Design review of the part built by this model. Coordinates are the model's own, in mm. A direction names the side the tool comes from. Coordinates: 2 decimals unless noted, no trailing zeros. Order: outer loops, then holes, each group sorted by start corner. A loop starts at its lowest first (then second) coordinate and runs counter-clockwise, first axis right, second up. Notation, with made-up numbers: M 24,-40 L 51,-40 A14 cw 51,-35 Z; hole C -11,-17 d10. An arc over 180 degrees is marked long. Answer as a JSON object with one key per item and string values.
from build123d import *

# Parameters (mm, degrees)
SKETCH1_W           = 66
SKETCH1_H           = 180
BOSS_EXTRUDE1_DEPTH = 34.7
FILLET1_R           = 10
SHELL1_T            = -3.1
SKETCH4_R           = 6.5
CUT_EXTRUDE4_DEPTH  = 35.7
SKETCH2_R           = 3.25
CUT_EXTRUDE5_DEPTH  = 35.7
SKETCH5_W           = 27
SKETCH5_H           = 15.2
CUT_EXTRUDE6_DEPTH  = 35.7
SKETCH6_W           = 5
SKETCH6_H           = 5
CUT_EXTRUDE10_DEPTH = 35.7
SKETCH31_R          = 0.5
CUT_EXTRUDE11_DEPTH = 35.7
SKETCH3_W           = 37.2
SKETCH3_H           = 37.3
CUT_EXTRUDE14_DEPTH = 2
SKETCH32_W          = 26.5
SKETCH32_H          = 15
CUT_EXTRUDE16_DEPTH = 5


with BuildPart() as part:
    # Sketch1 → Boss-Extrude1 (new body)
    with BuildSketch(Plane(origin=(0, 0, 0), x_dir=(1, 0, 0), z_dir=(0, 1, 0))):
        with Locations((33, 90)):
            Rectangle(SKETCH1_W, SKETCH1_H)
    extrude(amount=BOSS_EXTRUDE1_DEPTH)

    # Fillet1
    fillet1_edges = [part.edges().sort_by_distance(p)[0] for p in [
        (66, 34.7, -90),
        (0, 34.7, -90),
    ]]
    fillet(fillet1_edges, radius=FILLET1_R)

    # Shell1
    shell1_openings = [part.faces().sort_by_distance(p)[0] for p in [
        (33, 0, -90),
    ]]
    offset(amount=SHELL1_T, openings=shell1_openings, kind=Kind.INTERSECTION)

    # Sketch4 → Cut-Extrude4 (cut, through all)
    with BuildSketch(Plane(origin=(0, 34.7, 0), x_dir=(1, 0, 0), z_dir=(0, 1, 0))):
        with Locations((48.1, 89.6)):
            Circle(SKETCH4_R)
        with Locations((17.9, 89.6)):
            Circle(SKETCH4_R)
    extrude(amount=-CUT_EXTRUDE4_DEPTH, mode=Mode.SUBTRACT)

    # Sketch2 → Cut-Extrude5 (cut, through all)
    with BuildSketch(Plane(origin=(0, 34.7, 0), x_dir=(1, 0, 0), z_dir=(0, 1, 0))):
        with Locations((33, 64.3)):
            Circle(SKETCH2_R)
    extrude(amount=-CUT_EXTRUDE5_DEPTH, mode=Mode.SUBTRACT)

    # Sketch5 → Cut-Extrude6 (cut, through all)
    with BuildSketch(Plane(origin=(0, 34.7, 0), x_dir=(1, 0, 0), z_dir=(0, 1, 0))):
        with Locations((33, 117.9)):
            Rectangle(SKETCH5_W, SKETCH5_H)
    extrude(amount=-CUT_EXTRUDE6_DEPTH, mode=Mode.SUBTRACT)

    # Sketch6 → Cut-Extrude10 (cut, through all)
    with BuildSketch(Plane(origin=(0, 34.7, 0), x_dir=(1, 0, 0), z_dir=(0, 1, 0))):
        with Locations((50, 148.979436507)):
            Rectangle(SKETCH6_W, SKETCH6_H)
        with Locations((16, 148.979436507)):
            Rectangle(SKETCH6_W, SKETCH6_H)
    extrude(amount=-CUT_EXTRUDE10_DEPTH, mode=Mode.SUBTRACT)

    # Sketch31 → Cut-Extrude11 (cut, through all)
    with BuildSketch(Plane(origin=(0, 34.7, 0), x_dir=(1, 0, 0), z_dir=(0, 1, 0))):
        with Locations((28.628571429, 166.273512362)):
            Circle(SKETCH31_R)
        with Locations((30.028571429, 166.273512362)):
            Circle(SKETCH31_R)
        with Locations((31.428571429, 166.273512362)):
            Circle(SKETCH31_R)
        with Locations((32.828571429, 166.273512362)):
            Circle(SKETCH31_R)
        with Locations((34.228571429, 166.273512362)):
            Circle(SKETCH31_R)
        with Locations((35.628571429, 166.273512362)):
            Circle(SKETCH31_R)
        with Locations((37.028571429, 166.273512362)):
            Circle(SKETCH31_R)
        with Locations((30.028571429, 164.873512362)):
            Circle(SKETCH31_R)
        with Locations((31.428571429, 164.873512362)):
            Circle(SKETCH31_R)
        with Locations((32.828571429, 164.873512362)):
            Circle(SKETCH31_R)
        with Locations((34.228571429, 164.873512362)):
            Circle(SKETCH31_R)
        with Locations((35.628571429, 164.873512362)):
            Circle(SKETCH31_R)
        with Locations((37.028571429, 164.873512362)):
            Circle(SKETCH31_R)
        with Locations((30.028571429, 163.473512362)):
            Circle(SKETCH31_R)
        with Locations((31.428571429, 163.473512362)):
            Circle(SKETCH31_R)
        with Locations((32.828571429, 163.473512362)):
            Circle(SKETCH31_R)
        with Locations((34.228571429, 163.473512362)):
            Circle(SKETCH31_R)
        with Locations((35.628571429, 163.473512362)):
            Circle(SKETCH31_R)
        with Locations((37.028571429, 163.473512362)):
            Circle(SKETCH31_R)
        with Locations((30.028571429, 162.073512362)):
            Circle(SKETCH31_R)
        with Locations((31.428571429, 162.073512362)):
            Circle(SKETCH31_R)
        with Locations((32.828571429, 162.073512362)):
            Circle(SKETCH31_R)
        with Locations((34.228571429, 162.073512362)):
            Circle(SKETCH31_R)
        with Locations((35.628571429, 162.073512362)):
            Circle(SKETCH31_R)
        with Locations((37.028571429, 162.073512362)):
            Circle(SKETCH31_R)
        with Locations((30.028571429, 160.673512362)):
            Circle(SKETCH31_R)
        with Locations((31.428571429, 160.673512362)):
            Circle(SKETCH31_R)
        with Locations((32.828571429, 160.673512362)):
            Circle(SKETCH31_R)
        with Locations((34.228571429, 160.673512362)):
            Circle(SKETCH31_R)
        with Locations((35.628571429, 160.673512362)):
            Circle(SKETCH31_R)
        with Locations((37.028571429, 160.673512362)):
            Circle(SKETCH31_R)
        with Locations((30.028571429, 159.273512362)):
            Circle(SKETCH31_R)
        with Locations((31.428571429, 159.273512362)):
            Circle(SKETCH31_R)
        with Locations((32.828571429, 159.273512362)):
            Circle(SKETCH31_R)
        with Locations((34.228571429, 159.273512362)):
            Circle(SKETCH31_R)
        with Locations((35.628571429, 159.273512362)):
            Circle(SKETCH31_R)
        with Locations((37.028571429, 159.273512362)):
            Circle(SKETCH31_R)
        with Locations((30.028571429, 157.873512362)):
            Circle(SKETCH31_R)
        with Locations((31.428571429, 157.873512362)):
            Circle(SKETCH31_R)
        with Locations((32.828571429, 157.873512362)):
            Circle(SKETCH31_R)
        with Locations((34.228571429, 157.873512362)):
            Circle(SKETCH31_R)
        with Locations((35.628571429, 157.873512362)):
            Circle(SKETCH31_R)
        with Locations((37.028571429, 157.873512362)):
            Circle(SKETCH31_R)
        with Locations((30.028571429, 156.473512362)):
            Circle(SKETCH31_R)
        with Locations((31.428571429, 156.473512362)):
            Circle(SKETCH31_R)
        with Locations((32.828571429, 156.473512362)):
            Circle(SKETCH31_R)
        with Locations((34.228571429, 156.473512362)):
            Circle(SKETCH31_R)
        with Locations((35.628571429, 156.473512362)):
            Circle(SKETCH31_R)
        with Locations((37.028571429, 156.473512362)):
            Circle(SKETCH31_R)
        with Locations((30.028571429, 155.073512362)):
            Circle(SKETCH31_R)
        with Locations((31.428571429, 155.073512362)):
            Circle(SKETCH31_R)
        with Locations((32.828571429, 155.073512362)):
            Circle(SKETCH31_R)
        with Locations((34.228571429, 155.073512362)):
            Circle(SKETCH31_R)
        with Locations((35.628571429, 155.073512362)):
            Circle(SKETCH31_R)
        with Locations((37.028571429, 155.073512362)):
            Circle(SKETCH31_R)
        with Locations((30.028571429, 153.673512362)):
            Circle(SKETCH31_R)
        with Locations((31.428571429, 153.673512362)):
            Circle(SKETCH31_R)
        with Locations((32.828571429, 153.673512362)):
            Circle(SKETCH31_R)
        with Locations((34.228571429, 153.673512362)):
            Circle(SKETCH31_R)
        with Locations((35.628571429, 153.673512362)):
            Circle(SKETCH31_R)
        with Locations((37.028571429, 153.673512362)):
            Circle(SKETCH31_R)
        with Locations((28.628571429, 164.873512362)):
            Circle(SKETCH31_R)
        with Locations((28.628571429, 163.473512362)):
            Circle(SKETCH31_R)
        with Locations((28.628571429, 162.073512362)):
            Circle(SKETCH31_R)
        with Locations((28.628571429, 160.673512362)):
            Circle(SKETCH31_R)
        with Locations((28.628571429, 159.273512362)):
            Circle(SKETCH31_R)
        with Locations((28.628571429, 157.873512362)):
            Circle(SKETCH31_R)
        with Locations((28.628571429, 156.473512362)):
            Circle(SKETCH31_R)
        with Locations((28.628571429, 155.073512362)):
            Circle(SKETCH31_R)
        with Locations((28.628571429, 153.673512362)):
            Circle(SKETCH31_R)
    extrude(amount=-CUT_EXTRUDE11_DEPTH, mode=Mode.SUBTRACT)

    # Sketch3 → Cut-Extrude14 (cut)
    with BuildSketch(Plane(origin=(0, 34.7, 0), x_dir=(1, 0, 0), z_dir=(0, 1, 0))):
        with Locations((33, 20.740021927)):
            Rectangle(SKETCH3_W, SKETCH3_H)
    extrude(amount=-CUT_EXTRUDE14_DEPTH, mode=Mode.SUBTRACT)

    # Sketch32 → Cut-Extrude16 (cut)
    with BuildSketch(Plane.XY):
        with Locations((33, 17.35)):
            Rectangle(SKETCH32_W, SKETCH32_H)
    extrude(amount=-CUT_EXTRUDE16_DEPTH, mode=Mode.SUBTRACT)


solid = part.part
1) Add section C-C (z = -64.3). State the section outline as (x, y) points, and give its area (3 significant figures).
Taken from the geometry:
{"outline": "M 0,0 L 3.1,0 L 3.1,24.7 A6.9 cw 10,31.6 L 29.75,31.6 L 29.75,34.7 L 10,34.7 A10 ccw 0,24.7 Z; M 36.25,31.6 L 56,31.6 A6.9 cw 62.9,24.7 L 62.9,0 L 66,0 L 66,24.7 A10 ccw 56,34.7 L 36.25,34.7 Z", "area": "358 mm2"}
2) Insertion check: pin 1 Ø0.9 at (y, z) = (32.5, -149.5) entering from +X; pin 2 Ø3.5 at (y, z) = (33, -115) entering from -X; pin 3 Ø1.6 at (y, z) = (33, -150) entering from -X; pin 4 Ø2.5 at (x, y) = (27.5, 33) entering from +Z. Each pin has a flat end and moves straight along its axis. Give the tip position at first contact, or say it passes through.
Taken from the geometry:
{"pin 1": "stops at x = 62.78", "pin 2": "stops at x = 2.44", "pin 3": "stops at x = 3.39", "pin 4": "stops at z = 0"}
3) Add section B-B (z = -149.5). State the section outline as (x, y) points.
Taken from the geometry:
{"outline": "M 0,0 L 3.1,0 L 3.1,24.7 A6.9 cw 10,31.6 L 13.5,31.6 L 13.5,34.7 L 10,34.7 A10 ccw 0,24.7 Z; M 18.5,31.6 L 47.5,31.6 L 47.5,34.7 L 18.5,34.7 Z; M 52.5,31.6 L 56,31.6 A6.9 cw 62.9,24.7 L 62.9,0 L 66,0 L 66,24.7 A10 ccw 56,34.7 L 52.5,34.7 Z"}
4) Tool access review of faces 5 (the flat face through (33, 32.7, -21)), 6 (the flat face through (52.5, 33, -149)), 7 (the cylindrical face through (5.07, 29.53, -91.22)): name each direction out of +Z, -Z, +X, -X, +Y, -Y from which nothing blocks a thin tool from reaching the whole face with its end or side.
Taken from the geometry:
{"face 5": "+Y", "face 6": "+Y, -Y", "face 7": "-Y"}
5) Add section D-D (z = -30.5). State the section outline as (x, y) points.
Taken from the geometry:
{"outline": "M 0,0 L 3.1,0 L 3.1,24.7 A6.9 cw 10,31.6 L 56,31.6 A6.9 cw 62.9,24.7 L 62.9,0 L 66,0 L 66,24.7 A10 ccw 56,34.7 L 51.6,34.7 L 51.6,32.7 L 14.4,32.7 L 14.4,34.7 L 10,34.7 A10 ccw 0,24.7 Z"}
6) Add section A-A (z = -122). State the section outline as (x, y) points, and give its area (3 significant figures).
Taken from the geometry:
{"outline": "M 0,0 L 3.1,0 L 3.1,24.7 A6.9 cw 10,31.6 L 19.5,31.6 L 19.5,34.7 L 10,34.7 A10 ccw 0,24.7 Z; M 46.5,31.6 L 56,31.6 A6.9 cw 62.9,24.7 L 62.9,0 L 66,0 L 66,24.7 A10 ccw 56,34.7 L 46.5,34.7 Z", "area": "294 mm2"}
7) To check wall thickness, follow L1, parallel to Z at x = 16.5, y = 10; L2, parallel to X at y = 18, z = -135.5; L3, parallel to Y at x = 40, z = -12. State the ranges of each line that lie inside material, in increasing order.
Taken from the geometry:
{"L1": "z = -180 to -176.9, -3.1 to 0", "L2": "x = 0 to 3.1, 62.9 to 66", "L3": "y = 31.6 to 32.7"}
8) Mouldability with a two-part tool opening along Z and no side actions: class faces 1 (the cylindrical face through (16.491, 33.172, -83.255)), 2 (the flat face through (33, 17, -180)), 3 (the flat face through (33, 24.85, -2)), 4 (the flat face through (18.5, 33, -149)) as released by +Z, released by -Z, zero draft, split by the parting line, or undercut.
Taken from the geometry:
{"face 1": "undercut", "face 2": "released by -Z", "face 3": "zero draft", "face 4": "undercut"}
